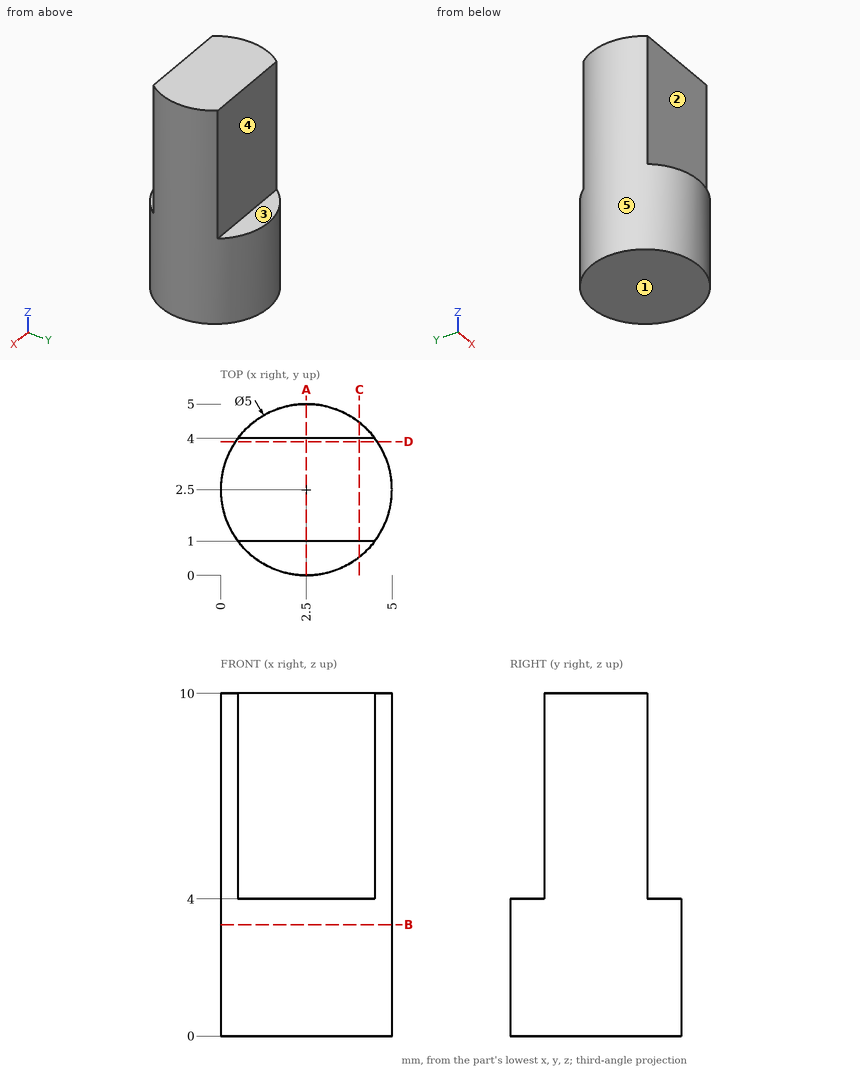
Here's the drawing with two shaded views (mm, measured from the low corner). I have some questions. A direction names the side the tool comes from. Give positions to 0.01 mm unless a question says otherwise; leave off trailing zeros. Write each loop counter-clockwise with the first axis right and the second up, starting at its lowest first coordinate (ties: lowest second). Pieces come first, ordered by that corner, then holes. Notation, with made-up numbers: (47, 35.25) -> (86, 35.25) arc R28 cw to (86, 60.25) -> close; hole circle Ø1 at (1.25, 57.25). An arc over 180 degrees is marked (long way). Use one line per item in the form item = value. Start each with the question number.
1. Imagine slicing it at D-D on y = 3.9. List the corners of the cut face in (x, z) for me.
2. Thinking about a two-plate mould opening in Z: for the marked faces 1, 2 and 3, which applies, +Z half, -Z half, draft (parallel to the pull), parting line (faces both ways), or undercut?
3. On a 3-axis mill with a long thin cutter (end or side, diameter ignored), from which of +Z, -Z, +X, -X, +Y, -Y can I reach the whole of each face in a straight line? I mean the marked faces 4 and 5. Say none if no direction works.
4. Imagine slicing it at C-C on x = 4.05. List the corners of the cut face in (y, z) for me.
5. Will these pins go through, and if not, where does the flat tip stop? pin 1 Ø3 at (x, z) = (3, 7) entering from +Y; pin 2 Ø1 at (y, z) = (4, 2) entering from +X; pin 3 Ø2 at (x, z) = (2, 8) entering from -Y.
6. Imagine slicing it at B-B on z = 3.25. List the corners of the cut face in (x, y) for me, plus the area to 3 significant figures.
7. Imagine slicing it at A-A on x = 2.5. List the corners of the cut face in (y, z) for me.
8. If I drill on L1, parallel to Z at x = 1.1, y = 0.95; L2, parallel to Y at x = 3.3, z = 8; L3, parallel to Y at x = 4, z = 1.75, over which ranges is the centre line in solid material (lowest first)?
Entries:
q1.outline = (0.43, 0) -> (4.57, 0) -> (4.57, 10) -> (0.43, 10) -> close
q2.face_1 = -Z half
q2.face_2 = draft
q2.face_3 = +Z half
q3.face_4 = +Z, +X, -X, +Y
q3.face_5 = +Z, -Z
q4.outline = (0.54, 0) -> (4.46, 0) -> (4.46, 4) -> (4, 4) -> (4, 10) -> (1, 10) -> (1, 4) -> (0.54, 4) -> close
q5.pin_1 = 4
q5.pin_2 = 4.79
q5.pin_3 = 1
q6.outline = circle Ø5 at (2.5, 2.5)
q6.area = 19.6 mm²
q7.outline = (0, 0) -> (5, 0) -> (5, 4) -> (4, 4) -> (4, 10) -> (1, 10) -> (1, 4) -> (0, 4) -> close
q8.L1 = 0 to 4
q8.L2 = 1 to 4
q8.L3 = 0.5 to 4.5
